Build history of the part. All positions in model axes, mm. Coordinates: 2 decimals unless noted, no trailing zeros. Order: outer loops, then holes, each group sorted by start corner. A loop starts at its lowest first (then second) coordinate and runs counter-clockwise, first axis right, second up. Notation, with made-up numbers: (48.25, -28.5) - (86.25, -28.5) arc R18 cw to (86.25, 3.5) - close; hole circle Ø8 at (33, 59). An arc over 180 degrees is marked (long way). Return JSON: item names as keys, results as strings.
from build123d import *

# Parameters (mm, degrees)
SKETCH_1_W          = 390
SKETCH_1_H          = 250
EXTRUDE_1_DEPTH     = 2
SKETCH_2_W          = 130
SKETCH_2_H          = 40
SKETCH_2_W_2        = 125
SKETCH_2_H_2        = 60
CUT_EXTRUDE_1_DEPTH = 5
CUT_EXTRUDE_2_DEPTH = 10
FILLET_1_R          = 5
SKETCH_4_R          = 1.5
SKETCH_4_R_2        = 1.75
CUT_EXTRUDE_3_DEPTH = 232.633330935


with BuildPart() as part:
    # 스케치1 → 보스-돌출1 (new body)
    with BuildSketch(Plane(origin=(0, 0, 0), x_dir=(1, 0, 0), z_dir=(0, 1, 0))):
        Rectangle(SKETCH_1_W, SKETCH_1_H)
    extrude(amount=EXTRUDE_1_DEPTH)

    # 스케치2 → 컷-돌출1 (cut)
    with BuildSketch(Plane(origin=(0, 2, 0), x_dir=(1, 0, 0), z_dir=(0, 1, 0))):
        with Locations((-85, 105)):
            Rectangle(SKETCH_2_W, SKETCH_2_H)
        with Locations((-85, -105)):
            Rectangle(SKETCH_2_W, SKETCH_2_H)
        with Locations((132.5, 95)):
            Rectangle(SKETCH_2_W_2, SKETCH_2_H_2)
        with Locations((132.5, -95)):
            Rectangle(SKETCH_2_W_2, SKETCH_2_H_2)
    extrude(amount=-CUT_EXTRUDE_1_DEPTH, mode=Mode.SUBTRACT)

    # 스케치3 → 컷-돌출2 (cut)
    with BuildSketch(Plane(origin=(0, 2, 0), x_dir=(1, 0, 0), z_dir=(0, 1, 0))):
        Polygon((-5, 125), (70, 65), (70, 125), align=None)
        Polygon((70, -65), (-5, -125), (70, -125), align=None)
    extrude(amount=-CUT_EXTRUDE_2_DEPTH, mode=Mode.SUBTRACT)

    # 필렛1
    fillet_1_edges = [part.edges().sort_by_distance(p)[0] for p in [
        (-5, 1, -125),
        (-5, 1, 125),
        (-150, 1, 125),
        (-20, 1, 125),
        (195, 1, -65),
        (195, 1, 65),
        (-150, 1, -125),
        (-20, 1, -125),
        (-195, 1, 125),
        (-195, 1, -125),
    ]]
    fillet(fillet_1_edges, radius=FILLET_1_R)

    # 스케치4 → 컷-돌출3 (cut, through all)
    with BuildSketch(Plane(origin=(0, 2, 0), x_dir=(1, 0, 0), z_dir=(0, 1, 0))):
        with Locations(Location((-100, 77, 0), (0, 0, 270))):
            Circle(SKETCH_4_R)
        with Locations(Location((-70, 77, 0), (0, 0, 270))):
            Circle(SKETCH_4_R)
        with Locations(Location((-70, 53, 0), (0, 0, 270))):
            Circle(SKETCH_4_R)
        with Locations(Location((-100, 53, 0), (0, 0, 270))):
            Circle(SKETCH_4_R)
        with Locations(Location((-100, -53, 0), (0, 0, 90))):
            Circle(SKETCH_4_R)
        with Locations(Location((-70, -53, 0), (0, 0, 90))):
            Circle(SKETCH_4_R)
        with Locations(Location((-70, -77, 0), (0, 0, 90))):
            Circle(SKETCH_4_R)
        with Locations(Location((-100, -77, 0), (0, 0, 90))):
            Circle(SKETCH_4_R)
        with Locations(Location((100, 60, 0), (0, 0, 270))):
            Circle(SKETCH_4_R_2)
        with Locations(Location((110, 60, 0), (0, 0, 270))):
            Circle(SKETCH_4_R_2)
        with Locations(Location((100, 10, 0), (0, 0, 270))):
            Circle(SKETCH_4_R_2)
        with Locations(Location((110, 10, 0), (0, 0, 270))):
            Circle(SKETCH_4_R_2)
        with Locations(Location((100, -10, 0), (0, 0, 270))):
            Circle(SKETCH_4_R_2)
        with Locations(Location((110, -10, 0), (0, 0, 270))):
            Circle(SKETCH_4_R_2)
        with Locations(Location((100, -60, 0), (0, 0, 270))):
            Circle(SKETCH_4_R_2)
        with Locations(Location((110, -60, 0), (0, 0, 270))):
            Circle(SKETCH_4_R_2)
    extrude(amount=-CUT_EXTRUDE_3_DEPTH, mode=Mode.SUBTRACT)


solid = part.part
1. Probe L1, parallel to X at y = 0.4, z = 53; L2, parallel to Z at x = -70, y = 0.95; L3, parallel to Z at x = 110, y = 0.85. List the from-to ranges inside material, lowest first.
Check values:
{"L1": "-195 to -101.5, -98.5 to -71.5, -68.5 to 195", "L2": "-85 to -78.5, -75.5 to -54.5, -51.5 to 51.5, 54.5 to 75.5, 78.5 to 85", "L3": "-65 to -61.75, -58.25 to -11.75, -8.25 to 8.25, 11.75 to 58.25, 61.75 to 65"}
2. Cut at B-B on x = -115. Give the cut face in (y, z), plus the area to 3 significant figures.
Check values:
{"outline": "(0, -85) - (2, -85) - (2, 85) - (0, 85) - close", "area": "340 mm²"}
3. Cut at A-A on y = 0.8. State how many separate pieces and enclosed holes the cut face has, plus the area to 3 significant figures.
Check values:
{"separate pieces": "1", "enclosed holes": "16", "area": "67,400 mm²"}
4. Drop flat-ended pins along their axis: pin 1 (1 mm diameter, centred on y = 1.5, z = -98.5, fed in from +X); pin 2 (4.5 mm diameter, centred on x = 110, z = 10, fed in from +Y); pin 3 (0.6 mm diameter, centred on x = -74.5, y = 1, fed in from -Z). Give the stop position or say it passes through.
Check values:
{"pin 1": "x = 28.75", "pin 2": "y = 2", "pin 3": "z = -85"}
